Check sheet for the modelled part. Datum: model origin and axes. Units: mm. A direction names the side the tool comes from. Give positions to 0.01 mm unless a question says otherwise; leave off trailing zeros. Write each loop counter-clockwise with the first axis right and the second up, starting at its lowest first coordinate (ties: lowest second). Pieces come first, ordered by that corner, then holes. Notation, with made-up numbers: (-0.75, 86.5) -> (37.25, 86.5) arc R23 ccw to (37.25, 98.5) -> close; hole circle Ø4 at (20.5, 87). An arc over 180 degrees is marked (long way). Return JSON: item names as keys, results as strings.
from build123d import *

# Parameters (mm, degrees)
SKETCH004_W   = 15
SKETCH004_H   = 60
SKETCH004_R   = 6
SKETCH004_W_2 = 8
SKETCH004_H_2 = 15
PAD004_DEPTH  = 2
SKETCH003_W   = 15
SKETCH003_H   = 60
PAD003_DEPTH  = 2
SKETCH002_W   = 90
SKETCH002_H   = 15
PAD002_DEPTH  = 2
SKETCH001_W   = 90
SKETCH001_H   = 15
PAD001_DEPTH  = 2
SKETCH_W      = 90
SKETCH_H      = 70
SKETCH_R      = 2.5
SKETCH_R_2    = 1.5
PAD_DEPTH     = 2


with BuildPart() as body004:
    # Sketch004 → Pad004 (new body)
    with BuildSketch(Plane.YZ):
        with Locations((7.5, 0)):
            Rectangle(SKETCH004_W, SKETCH004_H)
        with Locations((8, 15)):
            Circle(SKETCH004_R, mode=Mode.SUBTRACT)
        with Locations((9, -12.5)):
            Rectangle(SKETCH004_W_2, SKETCH004_H_2, mode=Mode.SUBTRACT)
    extrude(amount=PAD004_DEPTH)


with BuildPart() as body004_1:
    # Body004 placement: moved
    add(body004.part.moved(Location((43, 0, 0))))


with BuildPart() as body003:
    # Sketch003 → Pad003 (new body)
    with BuildSketch(Plane.YZ):
        with Locations((7.5, 0)):
            Rectangle(SKETCH003_W, SKETCH003_H)
    extrude(amount=PAD003_DEPTH)


with BuildPart() as body003_1:
    # Body003 placement: moved
    add(body003.part.moved(Location((-45, 0, 0))))


with BuildPart() as body002:
    # Sketch002 → Pad002 (new body)
    with BuildSketch(Plane.XY):
        with Locations((0, 7.5)):
            Rectangle(SKETCH002_W, SKETCH002_H)
    extrude(amount=PAD002_DEPTH)


with BuildPart() as body002_1:
    # Body002 placement: moved
    add(body002.part.moved(Location((0, 0, -30))))


with BuildPart() as body001:
    # Sketch001 → Pad001 (new body)
    with BuildSketch(Plane.XY):
        with Locations((0, 7.5)):
            Rectangle(SKETCH001_W, SKETCH001_H)
    extrude(amount=PAD001_DEPTH)


with BuildPart() as body001_1:
    # Body001 placement: moved
    add(body001.part.moved(Location((0, 0, 28))))


with BuildPart() as fusion003:
    # Sketch → Pad (new body)
    with BuildSketch(Plane.XZ):
        Rectangle(SKETCH_W, SKETCH_H)
        with Locations((-40, 25)):
            Circle(SKETCH_R, mode=Mode.SUBTRACT)
        with Locations((-40, -25)):
            Circle(SKETCH_R, mode=Mode.SUBTRACT)
        with Locations((40, -25)):
            Circle(SKETCH_R, mode=Mode.SUBTRACT)
        with Locations((40, 25)):
            Circle(SKETCH_R, mode=Mode.SUBTRACT)
        with Locations((-40, 32)):
            Circle(SKETCH_R_2, mode=Mode.SUBTRACT)
        with Locations((40, 32)):
            Circle(SKETCH_R_2, mode=Mode.SUBTRACT)
        with Locations((40, -32)):
            Circle(SKETCH_R_2, mode=Mode.SUBTRACT)
        with Locations((-40, -32)):
            Circle(SKETCH_R_2, mode=Mode.SUBTRACT)
    extrude(amount=PAD_DEPTH)

    # Fusion: union Body001
    add(body001_1.part)

    # Fusion001: union Body002
    add(body002_1.part)

    # Fusion002: union Body003
    add(body003_1.part)

    # Fusion003: union Body004
    add(body004_1.part)


solid = fusion003.part
(1) Cross-section at D-D on y = 9.75. Enter the section's corners in (x, z), then the cut area to 3 significant figures.
Reply:
{"outline": "(-45, -30) -> (45, -30) -> (45, -20) -> (43, -20) -> (43, -28) -> (-43, -28) -> (-43, 28) -> (43, 28) -> (43, 20.74) -> (45, 20.74) -> (45, 30) -> (-45, 30) -> close; (43, -5) -> (45, -5) -> (45, 9.26) -> (43, 9.26) -> close", "area": "531 mm^2"}
(2) Cross-section at A-A on x = 40. Enter the section's corners in (y, z).
Reply:
{"outline": "(-2, -35) -> (0, -35) -> (0, -33.5) -> (-2, -33.5) -> close; (-2, -30.5) -> (0, -30.5) -> (0, -30) -> (15, -30) -> (15, -28) -> (0, -28) -> (0, -27.5) -> (-2, -27.5) -> close; (-2, -22.5) -> (0, -22.5) -> (0, 22.5) -> (-2, 22.5) -> close; (-2, 27.5) -> (0, 27.5) -> (0, 28) -> (15, 28) -> (15, 30) -> (0, 30) -> (0, 30.5) -> (-2, 30.5) -> close; (-2, 33.5) -> (0, 33.5) -> (0, 35) -> (-2, 35) -> close"}
(3) Thickness scan on L1, parallel to Z at x = -40, y = -0.95; L2, parallel to Z at x = 43.6, y = 8; L3, parallel to X at y = 7.5, z = -4. Record the ranges inside material, lowest first.
Reply:
{"L1": "-35 to -33.5, -30.5 to -27.5, -22.5 to 22.5, 27.5 to 30.5, 33.5 to 35", "L2": "-30 to -20, -5 to 9, 21 to 30", "L3": "-45 to -43, 43 to 45"}
(4) Depth check by flat-ended pin: pin 1 Ø2.5 at (x, z) = (-5.5, -32.5) entering from +Y; pin 2 Ø4.5 at (x, y) = (-3, 4) entering from +Z; pin 3 Ø2 at (x, y) = (44, 8) entering from -Z. Enter the tip coordinate at first touch or a pass-through.
Reply:
{"pin 1": "y = 0", "pin 2": "z = 30", "pin 3": "z = -30"}
(5) Cross-section at B-B on z = -10.5. Enter the section's corners in (x, y), then the cut area to 3 significant figures.
Reply:
{"outline": "(-45, -2) -> (45, -2) -> (45, 5) -> (43, 5) -> (43, 0) -> (-43, 0) -> (-43, 15) -> (-45, 15) -> close; (43, 13) -> (45, 13) -> (45, 15) -> (43, 15) -> close", "area": "224 mm^2"}
(6) Release check for a two-part mould opening along Z. For faces 4 (the flat face through (45, 7, 0)), 5 (the cylindrical face through (-38.66, -0.99, 27.11)), 6 (the flat face through (-1, 8, -30)) record: pulls with the +Z half, pulls with the -Z half, needs draft (parallel to the pull), parting line crosses it, or undercut.
Reply:
{"face 4": "needs draft", "face 5": "undercut", "face 6": "pulls with the -Z half"}
(7) Cross-section at C-C on z = -32. Enter the section's corners in (x, y).
Reply:
{"outline": "(-45, -2) -> (-41.5, -2) -> (-41.5, 0) -> (-45, 0) -> close; (-38.5, -2) -> (38.5, -2) -> (38.5, 0) -> (-38.5, 0) -> close; (41.5, -2) -> (45, -2) -> (45, 0) -> (41.5, 0) -> close"}
(8) Set-up check for faces 1 (the flat face through (-1, 0, 33)), 2 (the flat face through (43, 7, 0)), 3 (the cylindrical face through (44, 2, 15)): record each of +Z, -Z, +X, -X, +Y, -Y from which the full face is reachable in a straight line by a thin tool's end or side.
Reply:
{"face 1": "+Z, +X, -X, +Y", "face 2": "+Y", "face 3": "+X"}
